Could you check a few things on this drawing? It's one solid part, dimensions in mm from its lowest x, y, z. A direction names the side the tool comes from. Round coordinates to 2 decimals unless told otherwise and drop trailing zeros. Write each loop counter-clockwise with the first axis right and the second up, starting at its lowest first coordinate (ties: lowest second). Pieces come first, ordered by that corner, then holes. Notation, with made-up numbers: (52.5, -3) - (74.5, -3) arc R23 ccw to (74.5, 26) - close; hole circle Ø9 at (37, -32.5). An arc over 180 degrees is marked (long way). Put each result on its own line as item: value.
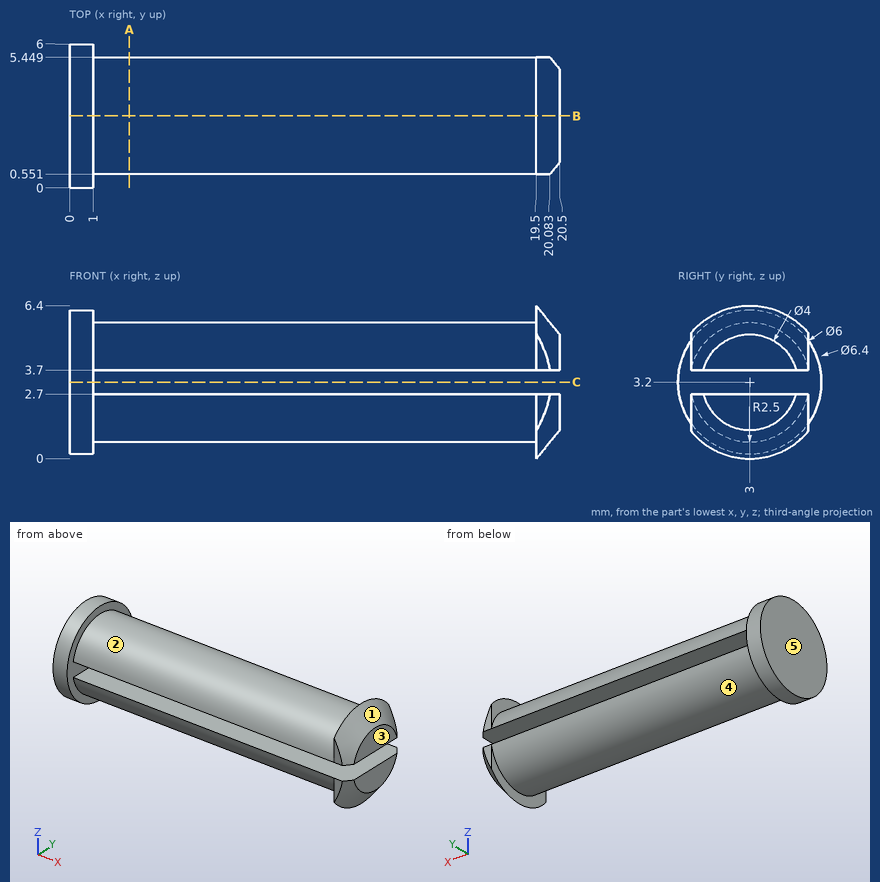
(1) Imagine slicing it at A-A, the plane x = 2.5. List the corners of the cut face in (y, z) for me.
Values found:
outline: (0.55, 2.7) arc R2.5 ccw to (5.45, 2.7) - close; (0.55, 3.7) - (5.45, 3.7) arc R2.5 ccw to start
(2) For the marked faces 1 and 2, which set-ups out of +Z, -Z, +X, -X, +Y, -Y let a thin tool reach every point of the face, with its end or its side?
Values found:
face 1: +Z, +X
face 2: +Z
(3) Please list where these lines run through material, in increasing order: probe 1 along Z at (x, y) = (12, 2.3); probe 2 along Z at (x, y) = (3.5, 4.75) (1 decimal); probe 3 along X at (y, z) = (1.55, 5.5). Write a range as from..to.
Values found:
probe 1: z = 0.8..2.7, 3.7..5.6
probe 2: z = 1.4..2.7, 3.7..5
probe 3: x = 0..1, 19.5..19.9
(4) Imagine slicing it at C-C, the plane z = 3.2. List the corners of the cut face in (x, y) for me.
Values found:
outline: (0, 0) - (1, 0) - (1, 6) - (0, 6) - close
(5) If we mould it in two halves opening along X, with no side actions, what happens to the marked faces 3, 4 and 5? For each: pulls with the +X half, pulls with the -X half, needs draft (parallel to the pull), parting line crosses it, or undercut.
Values found:
face 3: pulls with the +X half
face 4: undercut
face 5: pulls with the -X half
(6) Imagine slicing it at B-B, the plane y = 3. List the corners of the cut face in (x, z) for me.
Values found:
outline: (0, 0.2) - (1, 0.2) - (1, 0.7) - (19.5, 0.7) - (19.5, 0) - (20.5, 1.2) - (20.5, 2.7) - (1, 2.7) - (1, 3.7) - (20.5, 3.7) - (20.5, 5.2) - (19.5, 6.4) - (19.5, 5.7) - (1, 5.7) - (1, 6.2) - (0, 6.2) - close
(7) I'm going to push flat-ended pins straight in: pin 1 (0.5 mm diameter, centred on x = 19.5, z = 4.5, fed in from +Y); pin 2 (1.5 mm diameter, centred on x = 5.5, y = 4, fed in from -Z); pin 3 (0.8 mm diameter, centred on y = 3.5, z = 5.5, fed in from -X); pin 4 (2.5 mm diameter, centred on x = 14.5, y = 2.5, fed in from +Z). Where does each tip first touch, or does it pass through?
Values found:
pin 1: stops at y = 5.45
pin 2: stops at z = 0.71
pin 3: stops at x = 0
pin 4: stops at z = 5.7
